```python
from build123d import *

# Parameters (mm, degrees)
SKETCH_R     = 2.5
PAD_DEPTH    = 10
SKETCH001_W  = 9
SKETCH001_H  = 5.15
POCKET_DEPTH = 16
FILLET_R     = 0.5
FILLET001_R  = 1


with BuildPart() as part:
    # Sketch → Pad (new body)
    with BuildSketch(Plane.XY):
        Polygon((-15, 10), (-15, -10), (10, -3.5), (10, 3.5), align=None)
        Circle(SKETCH_R, mode=Mode.SUBTRACT)
    extrude(amount=PAD_DEPTH)

    # Sketch001 (on Face3 of Pad) → Pocket (cut)
    with BuildSketch(Plane.YZ.offset(10)):
        with Locations((0, 5)):
            Rectangle(SKETCH001_W, SKETCH001_H)
    extrude(amount=-POCKET_DEPTH, mode=Mode.SUBTRACT)

    # Fillet
    fillet_edges = [part.edges().sort_by_distance(p)[0] for p in [
        (-2.5, 6.75, 0),
        (-15, 10, 5),
        (-2.5, 6.75, 10),
        (10, 3.5, 8.7875),
        (8.076923, 4, 7.575),
        (6.153846, 4.5, 5),
        (8.076923, 4, 2.425),
        (10, 3.5, 1.2125),
        (-15, 0, 0),
        (-2.5, -6.75, 0),
        (10, 0, 0),
        (-2.5, 0, 0),
        (-15, -10, 5),
        (-15, 0, 10),
        (10, -3.5, 1.2125),
        (8.076923, -4, 2.425),
        (6.153846, -4.5, 5),
        (8.076923, -4, 7.575),
        (10, -3.5, 8.7875),
        (-2.5, -6.75, 10),
        (10, 0, 10),
        (-2.5, 0, 10),
        (10, 0, 7.575),
        (10, 0, 2.425),
    ]]
    fillet(fillet_edges, radius=FILLET_R)

    # Fillet001
    fillet001_edges = [part.edges().sort_by_distance(p)[0] for p in [
        (-6, 0, 7.575),
        (-6, 4.5, 5),
        (-6, 0, 2.425),
        (-6, -4.5, 5),
    ]]
    fillet(fillet001_edges, radius=FILLET001_R)


solid = part.part
```
Here's how the part is built. I have some questions about the finished solid (model axes, mm). A direction names the side the tool comes from. Coordinates: 2 decimals unless noted, no trailing zeros. Order: outer loops, then holes, each group sorted by start corner. A loop starts at its lowest first (then second) coordinate and runs counter-clockwise, first axis right, second up.
1) Which directions (+Z, -Z, +X, -X, +Y, -Y) give clear straight access to the entire face, cutting with the end or side of a thin tool? Please do faces 1 (the face through (-5.7, 0.06, 7.29)), 2 (the face through (6.013, 4.389, 2.275)), 3 (the face through (5.91, -4.42, 7.73)).
2) Imagine slicing it at C-C on z = 4.75. List the corners of the cut face in (x, y) for me, and give its area (3 significant figures).
3) Imagine slicing it at A-A on z = 1. List the corners of the cut face in (x, y) for me, and give its area (3 significant figures).
4) I need wall thicknesses on line 1 (X direction, y = 0, z = 8.7); line 2 (Y direction, x = 0, z = 8.7); line 3 (X direction, y = -5, z = 2.5). Which ranges of each line are inside material? Lowest first, please.
5) We'd pull the mould along Y, two halves only. Please class faces 4 (the face through (-2.242, -6.536, 9.85)), 5 (the face through (2.74, -4.95, 4.96)), 6 (the face through (10, 0, 1)), 7 (the face through (-6, 0, 5)): +Y half, -Y half, draft (parallel to the pull), parting line (faces both ways), or undercut.
6) Will these pins go through, and if not, where does the flat tip stop? pin 1 (10.5 mm diameter, centred on x = -0.5, y = -1, fed in from -Z); pin 2 (4 mm diameter, centred on x = 0, y = 0, fed in from +Z); pin 3 (1.6 mm diameter, centred on y = -1.5, z = 4.5, fed in from +X); pin 4 (1.5 mm diameter, centred on x = -3, z = 6, fed in from -Y) (3 decimals).
7) Imagine slicing it at B-B on y = 0. List the corners of the cut face in (x, z) for me (3 decimals), and give its area (3 significant figures).
8) Imagine slicing it at D-D on y = -2. State how many separate pieces and enclosed holes the cut face has, and give its area (3 significant figures).
Response values:
1. face 1: +X
1. face 2: +X, +Y
1. face 3: +X, -Y
2. outline: (-15, -9.35) arc R0.5 ccw to (-14.37, -9.84) - (2.37, -5.48) arc R0.5 ccw to (2.24, -4.5) - (-5, -4.5) arc R1 cw to (-6, -3.5) - (-6, 3.5) arc R1 cw to (-5, 4.5) - (2.24, 4.5) arc R0.5 ccw to (2.37, 5.48) - (-14.37, 9.84) arc R0.5 ccw to (-15, 9.35) - close
2. area: 194 mm2
3. outline: (-15, -9.35) arc R0.5 ccw to (-14.37, -9.84) - (9.63, -3.6) arc R0.5 ccw to (10, -3.11) - (10, 3.11) arc R0.5 ccw to (9.63, 3.6) - (-14.37, 9.84) arc R0.5 ccw to (-15, 9.35) - close; hole circle Ø5 at (0, 0)
3. area: 318 mm2
4. line 1: x = -15 to -2.5, 2.5 to 10
4. line 2: y = -6.1 to -2.5, 2.5 to 6.1
4. line 3: x = -15 to 2.74
5. face 4: -Y half
5. face 5: undercut
5. face 6: draft
5. face 7: undercut
6. pin 1: stops at z = 0
6. pin 2: passes through
6. pin 3: stops at x = -6
6. pin 4: stops at y = -7.075
7. outline: (-15, 0.5) arc R0.5 ccw to (-14.5, 0) - (-3, 0) arc R0.5 ccw to (-2.5, 0.5) - (-2.5, 2.425) - (-5, 2.425) arc R1 cw to (-6, 3.425) - (-6, 6.575) arc R1 cw to (-5, 7.575) - (-2.5, 7.575) - (-2.5, 9.5) arc R0.5 ccw to (-3, 10) - (-14.5, 10) arc R0.5 ccw to (-15, 9.5) - close; (2.5, 0.5) arc R0.5 ccw to (3, 0) - (9.5, 0) arc R0.5 ccw to (10, 0.5) - (10, 1.925) arc R0.5 ccw to (9.5, 2.425) - (2.5, 2.425) - close; (2.5, 7.575) - (9.5, 7.575) arc R0.5 ccw to (10, 8.075) - (10, 9.5) arc R0.5 ccw to (9.5, 10) - (3, 10) arc R0.5 ccw to (2.5, 9.5) - close
7. area: 143 mm2
8. separate pieces: 3
8. enclosed holes: 0
8. area: 153 mm2
